The listing builds one solid part. Answer for the finished solid, in the listing's coordinates (mm). A direction names the side the tool comes from. Give positions to 0.01 mm unless a question says otherwise; leave off trailing zeros. Loops run counter-clockwise (first coordinate to the right, second up) from the corner with the lowest first, then second, coordinate; pieces in that order, holes last.
Item 1: Each of these flat-tipped pins is pushed along its axis until it touches: pin 1 Ø2.5 at (y, z) = (-6, 5.5) entering from +X; pin 2 Ø1.5 at (x, y) = (-1, 23.5) entering from -Z; pin 3 Ø4 at (x, y) = (7, 9) entering from -Z; pin 4 Ø1 at (y, z) = (5, 10.5) entering from -X. Where does it stop, or does it pass through?
Item 2: The mould has two halves that part along Y. Classify faces 1 (the face through (-16.629, -5, 6)), 2 (the face through (3.371, 12, 11)), 3 (the face through (-6, -2.062, 6)), 4 (the face through (-6, -7.062, 6)): pulls with the +Y half, pulls with the -Y half, needs draft (parallel to the pull), parting line crosses it, or undercut.
Item 3: Section B-B, the plane z = 2.75 is taken. Give the vertices of the cut face in (x, y).
Item 4: Consider line 1 along Y through (x, z) = (-8, 1.5); line 2 along X through (y, z) = (-5, 5.75); line 3 along X through (y, z) = (20.5, 10.5). Determine where each line is inside the solid, lowest interval first.
Item 5: Section C-C, the plane y = -2.5 is taken. Give the vertices of the cut face in (x, z).
Item 6: Section D-D, the plane z = 9.5 is taken. Give the vertices of the cut face in (x, y).
Item 7: A tool of negligible diameter and unlimited length cuts with its end or side. For faces 5 (the face through (-7, -5, 0)), 6 (the face through (3.371, 28, 4)), from which of +Z, -Z, +X, -X, +Y, -Y can it reach the whole face along a straight path? Write none if from no direction.
Item 8: Section A-A, the plane x = -0.5 is taken. Give the vertices of the cut face in (y, z), and give its area (3 significant figures).
Autodesk Inventor part; units mm, degrees
ref_plane "YZ Plane" through (0, 0, 0) normal (1, 0, 0) x (0, 1, 0)
ref_plane "XZ Plane" through (0, 0, 0) normal (0, 1, 0) x (-1, 0, 0)
ref_plane "XY Plane" through (0, 0, 0) normal (0, 0, 1) x (1, 0, 0)
sketch "Sketch1" plane through (0, 0, 0) normal (0, 0, 1) x (1, 0, 0)
  line L0 (-16.6287, 30.9385) -> (3.3713, 30.9385)
  line L1 (3.3713, 30.9385) -> (3.3713, 25.9385)
  line L2 (3.3713, 25.9385) -> (-16.6287, 25.9385)
  line L3 (-16.6287, 25.9385) -> (-16.6287, 30.9385)
  line L4 (-16.6287, -2.0615) -> (3.3713, -2.0615)
  line L5 (3.3713, -2.0615) -> (3.3713, -7.0615)
  line L6 (3.3713, -7.0615) -> (-16.6287, -7.0615)
  line L7 (-16.6287, -7.0615) -> (-16.6287, -2.0615)
  point P0 (0, 0)
  dimension "d0" = 20
  dimension "d1" = 5
  dimension "d2" = 5
  dimension "d3" = 20
  dimension "d4" = 38
extrude "Extrusion1" add sketch "Sketch1" along normal blind 10
sketch "Sketch2" plane through (0, 0, 10) normal (0, 0, 1) x (1, 0, 0)
  line L0 (-16.6287, 30.9385) -> (8.3713, 30.9385)
  line L1 (8.3713, 30.9385) -> (8.3713, -7.0615)
  line L2 (8.3713, -7.0615) -> (-16.6287, -7.0615)
  line L3 (-16.6287, -7.0615) -> (-16.6287, 30.9385)
  line L4 (-16.6287, -7.0615) -> (3.3713, -7.0615)
  point P0 (0, 0)
  dimension "d7" = 25
extrude "Extrusion2" add sketch "Sketch2" along normal blind 1.2
fillet "Fillet1" radius 5 2 edges at (8.3713, 30.9385, 10.6) (8.3713, -7.0615, 10.6)
chamfer "Chamfer1" distance 2 angle 45 2 edges at (3.3713, -4.5615, 10) (3.3713, 28.4385, 10)
sketch "Sketch3" plane through (0, 0, 10) normal (0, 0, -1) x (-1, 0, 0)
  line L0 (16.6287, -2.0615) -> (-3.3713, -2.0615)
  line L1 (-3.3713, -2.0615) -> (-3.3713, 25.9385)
  line L2 (-3.3713, 25.9385) -> (16.6287, 25.9385)
  line L3 (16.6287, 25.9385) -> (16.6287, -2.0615)
  point P0 (0, 0)
extrude "Extrusion3" cut sketch "Sketch3" against normal blind 1.2
properties part number "Fuse Box Support"
Worked answers:
1. pin 1: stops at x = 3.37
1. pin 2: passes through
1. pin 3: stops at z = 10
1. pin 4: stops at x = 3.37
2. face 1: needs draft
2. face 2: undercut
2. face 3: undercut
2. face 4: pulls with the -Y half
3. outline: (-16.63, -7.06) - (3.37, -7.06) - (3.37, -2.06) - (-16.63, -2.06) - close; (-16.63, 25.94) - (3.37, 25.94) - (3.37, 30.94) - (-16.63, 30.94) - close
4. line 1: y = -7.06 to -2.06, 25.94 to 30.94
4. line 2: x = -16.63 to 3.37
4. line 3: x = 3.37 to 8.37
5. outline: (-16.63, 0) - (3.37, 0) - (3.37, 8) - (5.37, 10) - (8.35, 10) - (8.35, 11.2) - (-16.63, 11.2) - close
6. outline: (-16.63, -7.06) - (3.37, -7.06) arc R5 ccw to (4.87, -6.83) - (4.87, -2.06) - (-16.63, -2.06) - close; (-16.63, 25.94) - (4.87, 25.94) - (4.87, 30.71) arc R5 ccw to (3.37, 30.94) - (-16.63, 30.94) - close
7. face 5: -Z, +X, -X, +Y, -Y
7. face 6: -Z, +X, +Y, -Y
8. outline: (-7.06, 0) - (-2.06, 0) - (-2.06, 11.2) - (-7.06, 11.2) - close; (25.94, 0) - (30.94, 0) - (30.94, 11.2) - (25.94, 11.2) - close
8. area: 112 mm2
